Design review of the part built by this model. Coordinates are the model's own, in mm. A direction names the side the tool comes from. Give positions to 0.01 mm unless a question says otherwise; leave off trailing zeros. Write each loop counter-clockwise with the first axis right and the second up, starting at its lowest first coordinate (ties: lowest second). Pieces come first, ordered by that corner, then holes. Notation, with made-up numbers: M -17,18 L 32,18 A5 ccw 32,23 Z; hole C 2,75.25 d10. An arc over 180 degrees is marked long. Use a Markdown table: item, result. Add a question column.
```python
from build123d import *

# Parameters (mm, degrees)
SKETCH2_W            = 60
SKETCH2_H            = 85
BOSS_EXTRUDE1_DEPTH  = 5
BOSS_EXTRUDE2_DEPTH  = 20
BOSS_EXTRUDE3_DEPTH  = 20
FILLET1_R            = 10
FILLET2_R            = 5
FILLET3_R            = 12.5
FILLET1_OF_MIRROR1_R = 10
FILLET2_OF_MIRROR1_R = 5
FILLET3_OF_MIRROR1_R = 12.5
SKETCH4_R            = 5
CUT_EXTRUDE1_DEPTH   = 78.661122835
SKETCH5_R            = 2.75
CUT_EXTRUDE2_DEPTH   = 121.538251605
SKETCH6_R            = 2.75
CUT_EXTRUDE3_DEPTH   = 10


with BuildPart() as part:
    # Sketch2 → Boss-Extrude1 (new body)
    with BuildSketch(Plane(origin=(0, 0, 0), x_dir=(1, 0, 0), z_dir=(0, 1, 0))):
        with Locations((30, 0)):
            Rectangle(SKETCH2_W, SKETCH2_H)
    boss_extrude1 = extrude(amount=BOSS_EXTRUDE1_DEPTH)

    # Sketch3 → Boss-Extrude2 (add)
    with BuildSketch(Plane.XZ):
        Polygon((0, 25), (0, -25), (27.775312871, -25), (0.01, 0), (27.775312871, 25), align=None)
        Polygon((38.51, 0), (51.01, 11.255050554), (51.01, -11.255050554), align=None)
    boss_extrude2 = extrude(amount=BOSS_EXTRUDE2_DEPTH)

    # Sketch3_2 → Boss-Extrude3 (add)
    with BuildSketch(Plane.XZ):
        Polygon((0, 25), (0, -25), (27.775312871, -25), (0.01, 0), (27.775312871, 25), align=None)
        Polygon((38.51, 0), (51.01, 11.255050554), (51.01, -11.255050554), align=None)
    boss_extrude3 = extrude(amount=BOSS_EXTRUDE3_DEPTH)

    # Fillet1
    fillet1_edges = [part.edges().sort_by_distance(p)[0] for p in [
        (0.01, -10, 0),
    ]]
    fillet(fillet1_edges, radius=FILLET1_R)

    # Fillet2
    fillet2_edges = [part.edges().sort_by_distance(p)[0] for p in [
        (38.51, -10, 0),
    ]]
    fillet(fillet2_edges, radius=FILLET2_R)

    # Fillet3
    fillet3_edges = [part.edges().sort_by_distance(p)[0] for p in [
        (60, 2.5, -42.5),
        (60, 2.5, 42.5),
    ]]
    fillet(fillet3_edges, radius=FILLET3_R)

    # Mirror1: Boss-Extrude1, Boss-Extrude2, Boss-Extrude3 across plane
    add(boss_extrude1.mirror(Plane(origin=(0, 0, 0), x_dir=(0, 0, 1), z_dir=(1, 0, 0))))
    add(boss_extrude2.mirror(Plane(origin=(0, 0, 0), x_dir=(0, 0, 1), z_dir=(1, 0, 0))))
    add(boss_extrude3.mirror(Plane(origin=(0, 0, 0), x_dir=(0, 0, 1), z_dir=(1, 0, 0))))

    # Fillet1 of Mirror1
    fillet1_of_mirror1_edges = [part.edges().sort_by_distance(p)[0] for p in [
        (-0.01, -10, 0),
    ]]
    fillet(fillet1_of_mirror1_edges, radius=FILLET1_OF_MIRROR1_R)

    # Fillet2 of Mirror1
    fillet2_of_mirror1_edges = [part.edges().sort_by_distance(p)[0] for p in [
        (-38.51, -10, 0),
    ]]
    fillet(fillet2_of_mirror1_edges, radius=FILLET2_OF_MIRROR1_R)

    # Fillet3 of Mirror1
    fillet3_of_mirror1_edges = [part.edges().sort_by_distance(p)[0] for p in [
        (-60, 2.5, -42.5),
        (-60, 2.5, 42.5),
    ]]
    fillet(fillet3_of_mirror1_edges, radius=FILLET3_OF_MIRROR1_R)

    # Sketch4 → Cut-Extrude1 (cut, through all)
    with BuildSketch(Plane(origin=(0, 5, 0), x_dir=(1, 0, 0), z_dir=(0, 1, 0))):
        with Locations(Location((-50, 32.5, 0), (0, 0, 270))):
            Circle(SKETCH4_R)
        with Locations(Location((0, 32.5, 0), (0, 0, 270))):
            Circle(SKETCH4_R)
        with Locations(Location((51.276477942, 32.5, 0), (0, 0, 270))):
            Circle(SKETCH4_R)
        with Locations(Location((50, -32.5, 0), (0, 0, 270))):
            Circle(SKETCH4_R)
        with Locations(Location((0, -32.5, 0), (0, 0, 270))):
            Circle(SKETCH4_R)
        with Locations(Location((-50, -32.5, 0), (0, 0, 270))):
            Circle(SKETCH4_R)
        with BuildLine():
            Line((-32.5, 36.657579216), (-17.5, 36.657579216))
            ThreePointArc((-17.5, 36.657579216), (-13.342420784, 32.5), (-17.5, 28.342420784))
            Line((-17.5, 28.342420784), (-32.5, 28.342420784))
            ThreePointArc((-32.5, 28.342420784), (-36.657579216, 32.5), (-32.5, 36.657579216))
        make_face()
        with BuildLine():
            Line((17.5, 36.657579216), (32.5, 36.657579216))
            ThreePointArc((32.5, 36.657579216), (36.657579216, 32.5), (32.5, 28.342420784))
            Line((32.5, 28.342420784), (17.5, 28.342420784))
            ThreePointArc((17.5, 28.342420784), (13.342420784, 32.5), (17.5, 36.657579216))
        make_face()
        with BuildLine():
            Line((17.5, -27.766798153), (32.5, -27.766798153))
            ThreePointArc((32.5, -27.766798153), (37.233201847, -32.5), (32.5, -37.233201847))
            Line((32.5, -37.233201847), (17.5, -37.233201847))
            ThreePointArc((17.5, -37.233201847), (12.766798153, -32.5), (17.5, -27.766798153))
        make_face()
        with BuildLine():
            Line((-32.5, -28.155970988), (-17.5, -28.155970988))
            ThreePointArc((-17.5, -28.155970988), (-13.155970988, -32.5), (-17.5, -36.844029012))
            Line((-17.5, -36.844029012), (-32.5, -36.844029012))
            ThreePointArc((-32.5, -36.844029012), (-36.844029012, -32.5), (-32.5, -28.155970988))
        make_face()
        with BuildLine():
            Line((46.805058654, -20), (46.805058654, -12.5))
            ThreePointArc((46.805058654, -12.5), (50, -9.305058654), (53.194941346, -12.5))
            Line((53.194941346, -12.5), (53.194941346, -20))
            ThreePointArc((53.194941346, -20), (50, -23.194941346), (46.805058654, -20))
        make_face()
        with BuildLine():
            Line((53.389527763, 20), (53.389527763, 12.5))
            ThreePointArc((53.389527763, 12.5), (50, 9.110472237), (46.610472237, 12.5))
            Line((46.610472237, 12.5), (46.610472237, 20))
            ThreePointArc((46.610472237, 20), (50, 23.389527763), (53.389527763, 20))
        make_face()
        with BuildLine():
            Line((-46.62789073, 20), (-46.62789073, 12.5))
            ThreePointArc((-46.62789073, 12.5), (-50, 9.12789073), (-53.37210927, 12.5))
            Line((-53.37210927, 12.5), (-53.37210927, 20))
            ThreePointArc((-53.37210927, 20), (-50, 23.37210927), (-46.62789073, 20))
        make_face()
        with BuildLine():
            Line((-46.62789073, -12.5), (-46.62789073, -20))
            ThreePointArc((-46.62789073, -20), (-50, -23.37210927), (-53.37210927, -20))
            Line((-53.37210927, -20), (-53.37210927, -12.5))
            ThreePointArc((-53.37210927, -12.5), (-50, -9.12789073), (-46.62789073, -12.5))
        make_face()
    extrude(amount=-CUT_EXTRUDE1_DEPTH, mode=Mode.SUBTRACT)

    # Sketch5 → Cut-Extrude2 (cut, through all)
    with BuildSketch(Plane(origin=(51.01, 0, 0), x_dir=(0, 0, -1), z_dir=(1, 0, 0))):
        with Locations((0, -10.5)):
            Circle(SKETCH5_R)
    extrude(amount=-CUT_EXTRUDE2_DEPTH, mode=Mode.SUBTRACT)

    # Sketch6 → Cut-Extrude3 (cut)
    with BuildSketch(Plane.XZ):
        with Locations(Location((32, 12.5, 0), (0, 0, 270))):
            Circle(SKETCH6_R)
        with Locations(Location((24, 0, 0), (0, 0, 270))):
            Circle(SKETCH6_R)
        with Locations(Location((32, -12.5, 0), (0, 0, 270))):
            Circle(SKETCH6_R)
        with Locations(Location((-32, 12.5, 0), (0, 0, 270))):
            Circle(SKETCH6_R)
        with Locations(Location((-24, 0, 0), (0, 0, 270))):
            Circle(SKETCH6_R)
        with Locations(Location((-32, -12.5, 0), (0, 0, 270))):
            Circle(SKETCH6_R)
    extrude(amount=-CUT_EXTRUDE3_DEPTH, mode=Mode.SUBTRACT)


solid = part.part
```
(1) The part is to be moulded in two halves that separate along Y. For faces 1 (the cylindrical face through (46.063, -10.379, 2.747)), 2 (the flat face through (1, 5, -1)), 3 (the cylindrical face through (0.22, 2.535, 27.505)), say which applies: released by +Y, released by -Y, zero draft, split by the parting line, or undercut.
(2) Machinability: for faces 4 (the flat face through (-45.795, -9.86, -6.559)), 5 (the cylindrical face through (-36.843, 2.535, 32.596)), 6 (the flat face through (-51.01, -7.6, 0.1)), 7 (the cylindrical face through (-45.922, -7.773, 0.358)), 8 (the cylindrical face through (-5.1, -7.9, -1.7)), which of the approach directions +Z, -Z, +X, -X, +Y, -Y give a long, thin tool a straight path to every point of the face, cutting with its end or side? Answer none if there is none.
(3) For pin 1 (4.5 mm diameter, centred on x = -32, z = -12.5, fed in from -Y); pin 2 (2 mm diameter, centred on x = 22.5, y = -14.5, fed in from +Z); pin 3 (1.5 mm diameter, centred on y = -14, z = -6.5, fed in from +X); pin 4 (5.5 mm diameter, centred on y = -10, z = -1, fed in from -X), all flat-tipped, find the tip position at first contact; note any pin that passes through.
(4) Add section A-A on y = -3. Give the boundary of the cut face in (x, z).
(5) Add section B-B on x = 2. Give the boundary of the cut face in (y, z).
(6) Add section C-C on x = 16. Give the boundary of the cut face in (y, z), then the cut area to 3 significant figures.
(7) Add section D-D on z = 0. Give the number of separate pieces and of enclosed holes in the cut face, then the cut area to 3 significant figures.
(8) Wall thickness on L1, parallel to X at y = 3, z = -12.5; L2, parallel to Z at x = -6.5, y = -5.5; L3, parallel to Z at x = -47.5, y = 0.25: over which ranges is each line inside the solid? List them lowest first.
From the geometry:
| question | item | result |
|---|---|---|
| 1 | face 1 | undercut |
| 1 | face 2 | released by +Y |
| 1 | face 3 | zero draft |
| 2 | face 4 | -Z, -Y |
| 2 | face 5 | +Y, -Y |
| 2 | face 6 | +Z, -Z, -X, -Y |
| 2 | face 7 | +X, -X |
| 2 | face 8 | -Y |
| 3 | pin 1 | passes through |
| 3 | pin 2 | stops at z = 25 |
| 3 | pin 3 | stops at x = 51.01 |
| 3 | pin 4 | stops at x = -51.01 |
| 4 | outline | M -51.01,-9.28 A3.37 cw -48.87,-9.32 L -42.64,-3.72 A5 ccw -42.64,3.72 L -48.87,9.32 A3.37 cw -51.01,9.28 Z; M -27.78,-25 L 27.78,-25 L 8.26,-7.43 A10 cw 8.26,7.43 L 27.78,25 L -27.78,25 L -8.26,7.43 A10 cw -8.26,-7.43 Z; M 42.64,-3.72 L 48.85,-9.31 A3.39 cw 51.01,-9.26 L 51.01,9.47 A3.19 cw 49.02,9.46 L 42.64,3.72 A5 ccw Z |
| 5 | outline | M -20,-25 L 0,-25 L 0,-27.92 L 5,-27.92 L 5,27.92 L 0,27.92 L 0,25 L -20,25 Z; M 0,-42.5 L 5,-42.5 L 5,-37.08 L 0,-37.08 Z; M 0,37.08 L 5,37.08 L 5,42.5 L 0,42.5 Z; hole C -10.5,0 d5.5 |
| 6 | outline | M -20,-25 L 0,-25 L 0,-28.62 L 5,-28.62 L 5,28.01 L 0,28.01 L 0,25 L -20,25 L -20,14.4 L 0,14.4 L 0,-14.4 L -20,-14.4 Z; M 0,-42.5 L 5,-42.5 L 5,-36.38 L 0,-36.38 Z; M 0,36.99 L 5,36.99 L 5,42.5 L 0,42.5 Z |
| 6 | area | 765 mm^2 |
| 7 | separate pieces | 6 |
| 7 | enclosed holes | 0 |
| 7 | area | 979 mm^2 |
| 8 | L1 | x = -60 to -53.37, -46.63 to -34.75, -29.25 to 29.25, 34.75 to 46.61, 53.39 to 60 |
| 8 | L2 | z = -25 to -5.34, 5.34 to 25 |
| 8 | L3 | z = -42.5 to -36.83, -28.17 to -22.26, -10.24 to 10.24, 22.26 to 28.17, 36.83 to 42.5 |
